```python
from build123d import *

# Parameters (mm, degrees)
CROQUIS1_W              = 250
CROQUIS1_H              = 120
SALIENTE_EXTRUIR1_DEPTH = 60
SALIENTE_EXTRUIR2_DEPTH = 250
CROQUIS3_R              = 50
CORTAR_EXTRUIR1_DEPTH   = 5
CROQUIS5_R              = 30
CROQUIS5_R_2            = 20
CROQUIS5_W              = 15
CROQUIS5_H              = 70
CORTAR_EXTRUIR2_DEPTH   = 5


with BuildPart() as part:
    # Croquis1 → Saliente-Extruir1 (new body)
    with BuildSketch(Plane(origin=(0, 0, 0), x_dir=(1, 0, 0), z_dir=(0, 1, 0))):
        Rectangle(CROQUIS1_W, CROQUIS1_H)
    extrude(amount=SALIENTE_EXTRUIR1_DEPTH)

    # Croquis2 → Saliente-Extruir2 (add)
    with BuildSketch(Plane.ZY.offset(125)):
        Polygon((60, 60), (60, 0), (180, 0), (180, 30), align=None)
    extrude(amount=-SALIENTE_EXTRUIR2_DEPTH)

    # Croquis3 → Cortar-Extruir1 (cut)
    with BuildSketch(Plane(origin=(0, 60, 0), x_dir=(1, 0, 0), z_dir=(0, 1, 0))):
        with Locations(Location((0, 0, 0), (0, 0, 270))):
            Circle(CROQUIS3_R)
    extrude(amount=-CORTAR_EXTRUIR1_DEPTH, mode=Mode.SUBTRACT)

    # Croquis5 → Cortar-Extruir2 (cut)
    with BuildSketch(Plane(origin=(0, 70.588235294, 17.647058824), x_dir=(-1, 0, 0), z_dir=(0, 0.970142500145332, 0.24253562503633302))):
        with Locations(Location((80, 127.349581275, 0), (0, 0, 90))):
            Circle(CROQUIS5_R)
        with Locations(Location((80, 67.349581275, 0), (0, 0, 90))):
            Circle(CROQUIS5_R_2)
        with Locations(Location((37.573593129, 84.923174404, 0), (0, 0, 90))):
            Circle(CROQUIS5_R_2)
        with Locations(Location((20, 127.349581275, 0), (0, 0, 90))):
            Circle(CROQUIS5_R_2)
        with Locations(Location((-45, 87.349581275, 0), (0, 0, 90))):
            Circle(CROQUIS5_R_2)
        with Locations((-95, 105.502996891)):
            Rectangle(CROQUIS5_W, CROQUIS5_H)
    extrude(amount=-CORTAR_EXTRUIR2_DEPTH, mode=Mode.SUBTRACT)


solid = part.part
```
Work out the finished part from the listing and answer in its coordinate system (mm). A direction names the side the tool comes from. Round coordinates to 2 decimals unless told otherwise and drop trailing zeros. Loops run counter-clockwise (first coordinate to the right, second up) from the corner with the lowest first, then second, coordinate; pieces in that order, holes last. Notation, with made-up numbers: (-2, -16.5) -> (34, -16.5) arc R12 cw to (34, 1.5) -> close; hole circle Ø3 at (63, -9.75). An arc over 180 degrees is marked (long way). Write each question's results on one line, items separated by ' | '. Start each with the question number.
1. Section C-C (z = 33.5) is taken. Determine the outline of the cut face in (x, y).
2. Section B-B (x = 74) is taken. Determine the outline of the cut face in (y, z), plus the area to 3 significant figures.
3. For a pull along Y with two mould halves and no side action, classify faces 1 (the face through (-2, 0, 58)), 2 (the face through (1, 55, -1)), 3 (the face through (58.517, 50.587, 87.49)) as +Y half, -Y half, draft (parallel to the pull), parting line (faces both ways), or undercut.
4. A tool of negligible diameter and unlimited length cuts with its end or side. For faces 4 (the face through (-70.989, 30.37, 168.357)), 5 (the face through (15.02, 57.54, 47.69)), from which of +Z, -Z, +X, -X, +Y, -Y can it reach the whole face along a straight path? Write none if from no direction.
5. Given pin 1 Ø10 at (x, z) = (12, -0.5) entering from +Y, flat-ended and moving along its own axis, determine where the tip first touches the part or whether it passes through.
6. Section D-D (x = -75) is taken. Determine the outline of the cut face in (y, z), plus the area to 3 significant figures.
7. Section A-A (z = 0) is taken. Determine the outline of the cut face in (x, y), plus the area to 3 significant figures.
8. Find the intervals of material crossed by probe 1 along X at (y, z) = (57.65, 0); probe 2 along Y at (x, z) = (33.5, -23.5); probe 3 along Z at (x, y) = (88.5, 52), in increasing order. Write a range as from..to.
Evaluation:
1) outline: (-125, 0) -> (125, 0) -> (125, 60) -> (37.12, 60) -> (37.12, 55) -> (-37.12, 55) -> (-37.12, 60) -> (-125, 60) -> close
2) outline: (0, -60) -> (60, -60) -> (60, 60) -> (30, 180) -> (0, 180) -> close | area: 12,600 mm2
3) face 1: -Y half | face 2: +Y half | face 3: undercut
4) face 4: none | face 5: +Y
5) pin 1: stops at y = 55
6) outline: (0, -60) -> (60, -60) -> (60, 60) -> (58.95, 64.2) -> (54.1, 62.99) -> (44.71, 100.56) -> (49.56, 101.77) -> (46.88, 112.5) -> (42.03, 111.28) -> (27.68, 168.68) -> (32.53, 169.89) -> (30, 180) -> (0, 180) -> close | area: 12,100 mm2
7) outline: (-125, 0) -> (125, 0) -> (125, 60) -> (50, 60) -> (50, 55) -> (-50, 55) -> (-50, 60) -> (-125, 60) -> close | area: 14,500 mm2
8) probe 1: x = -125..-50, 50..125 | probe 2: y = 0..55 | probe 3: z = -60..85.67
